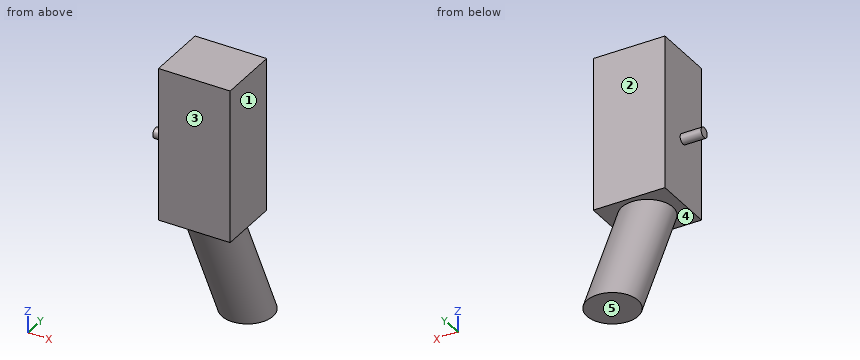
```python
from build123d import *

# Parameters (mm, degrees)
F0_W     = 70
F0_H     = 60
F1_DEPTH = 150
F3_R     = 25
F6_R     = 5
F7_DEPTH = 20.5


with BuildPart() as f1:
    # F0 (on Top) → F1 (new body)
    with BuildSketch(Plane.XY):
        with Locations((35, 30)):
            Rectangle(F0_W, F0_H)
    extrude(amount=F1_DEPTH)

    # F5: sweep along a path in F4
    with BuildLine(Plane.YZ.offset(35)) as f5_path:
        Line((29.8517439514, 0), (87.0807096362, -122.8410974145))
    # F3 (on face) → F5 (sweep)
    with BuildSketch(Plane(origin=(0, 0, 0), x_dir=(1, 0, 0), z_dir=(0, 0, -1))):
        with Locations((35, -30)):
            Circle(F3_R)
    sweep(path=f5_path.line)

    # F6 (on face) → F7 (join)
    with BuildSketch(Plane(origin=(0, 0, 0), x_dir=(0, -1, 0), z_dir=(-1, 0, 0))):
        with Locations((-30, 63.9334544539)):
            Circle(F6_R)
    extrude(amount=F7_DEPTH)


solid = f1.part
```
CAD build for the part. Positions are in the model's coordinates, mm. Face numbers are marked on the shaded views. A direction names the side the tool comes from. Round coordinates to 2 decimals unless told otherwise and drop trailing zeros. Order: outer loops, then holes, each group sorted by start corner. A loop starts at its lowest first (then second) coordinate and runs counter-clockwise, first axis right, second up. Notation, with made-up numbers: (27, 28) -> (77, 28) arc R29 cw to (77, 65) -> close; hole circle Ø6 at (49.25, 54). An arc over 180 degrees is marked (long way). Write item = value, one per line.
(1) Cut at A-A (z = 109). Write the cut outline in (x, y), plus the area to 3 significant figures.
Answers follow:
outline = (0, 0) -> (70, 0) -> (70, 60) -> (0, 60) -> close
area = 4,200 mm²
(2) Cut at B-B (x = 4). Write the cut outline in (y, z), plus the area to 3 significant figures.
Answers follow:
outline = (0, 0) -> (60, 0) -> (60, 150) -> (0, 150) -> close
area = 9,000 mm²
(3) 3-axis set-ups, long thin cutter, end or side, ignore diameter. For the marked faces 1 and 2: which of +Z, -Z, +X, -X, +Y, -Y reach the whole face in a straight line?
Answers follow:
face_1 = +Z, -Z, +X, +Y, -Y
face_2 = +Z, +X, -X, +Y
(4) Pull direction Z, two halves, no side cores. Call the marked faces 3, 4 and 5: +Z half, -Z half, draft (parallel to the pull), parting line (faces both ways), or undercut.
Answers follow:
face_3 = draft
face_4 = undercut
face_5 = -Z half
(5) Drill centre lines: L1, parallel to X at y = 12, z = 16; L2, parallel to Z at x = 63.5, y = 45.5; L3, parallel to Y at x = 54.5, z = 138.5. Where is each one in solid material? Low to high.
Answers follow:
L1 = 0 to 70
L2 = 0 to 150
L3 = 0 to 60
